Work out the finished part from the listing and answer in its coordinate system (mm). A direction names the side the tool comes from. Round coordinates to 2 decimals unless told otherwise and drop trailing zeros. Order: outer loops, then holes, each group sorted by start corner. A loop starts at its lowest first (then second) coordinate and runs counter-clockwise, first axis right, second up. Notation, with made-up numbers: (-9, 32) - (50, 32) arc R20 cw to (50, 67) - close; hole circle Ø4 at (-23, 75). An arc over 180 degrees is marked (long way). Use one line per item in the form item = value. Start each with the question number.
Q1. The part is cut by section D-D on z = 21.65. Determine the outline of the cut face in (x, y).
Q2. The part is cut by section B-B on y = 14. Determine the outline of the cut face in (x, z), plus the area to 3 significant figures.
Q3. The part is cut by section C-C on x = -15.65. Determine the outline of the cut face in (y, z), plus the area to 4 significant figures.
Q4. Given P1, Ø22.5, axis at x = 15, z = 10, coming from the +Y side; P2, Ø1, axis at x = -21.5, y = 17.5, coming from the +Z side; P3, Ø1.5, axis at x = -20, z = -4.5, coming from the -Y side, each flat-ended and moving along its own axis, determine where each tip first touches the part or whether it passes through.
Q5. Which of the six approach directions +Z, -Z, +X, -X, +Y, -Y give full straight-line access (tool end or side, diameter ignored) to faces 4 (the cylindrical face through (-17, 7, -9)), 5 (the flat face through (0, 35, -16.5))?
Q6. Find the intervals of material crossed by line 1 (Z direction, x = -15.65, y = 10.5); line 2 (X direction, y = 7.5, z = 22); line 3 (X direction, y = 9, z = -9), in increasing order. Write a range as [from, to].
Q7. For a pull along X with two mould halves and no side action, classify faces 1 (the cylindrical face through (15.325, 7.395, 20.186)), 2 (the flat face through (0, 7, 28.5)), 3 (the flat face through (32.5, 9, -7)) as +X half, -X half, draft (parallel to the pull), parting line (faces both ways), or undercut.
Q8. The part is cut by section A-A on z = 6. Determine the outline of the cut face in (x, y), plus the area to 3 significant figures.
from build123d import *

# Parameters (mm, degrees)
F0_W      = 65
F0_H      = 57
F1_DEPTH  = 55
F2_W      = 65
F2_H      = 45
F3_DEPTH  = 40
F4_R      = 11
F5_DEPTH  = 15
F6_R      = 1.5
F10_DEPTH = 15
F7_R      = 1.5
F11_DEPTH = 15
F8_R      = 1.5
F12_DEPTH = 15
F9_R      = 1.5
F13_DEPTH = 15


with BuildPart() as f1:
    # F0 (on Front) → F1 (new body)
    with BuildSketch(Plane.XZ):
        Rectangle(F0_W, F0_H)
    extrude(amount=-F1_DEPTH)

    # F2 (on face) → F3 (cut)
    with BuildSketch(Plane(origin=(0, 55, 0), x_dir=(-1, 0, 0), z_dir=(0, 1, 0))):
        with Locations((0, 6)):
            Rectangle(F2_W, F2_H)
    extrude(amount=-F3_DEPTH, mode=Mode.SUBTRACT)

    # F4 (on face) → F5 (cut)
    with BuildSketch(Plane.XZ):
        with Locations((0, 6)):
            Circle(F4_R)
    extrude(amount=-F5_DEPTH, mode=Mode.SUBTRACT)

    # F6 (on face) → F10 (cut)
    with BuildSketch(Plane.XZ):
        with Locations((15.65, 21.65)):
            Circle(F6_R)
    extrude(amount=-F10_DEPTH, mode=Mode.SUBTRACT)

    # F7 (on face) → F11 (cut)
    with BuildSketch(Plane.XZ):
        with Locations((-15.65, 21.65)):
            Circle(F7_R)
    extrude(amount=-F11_DEPTH, mode=Mode.SUBTRACT)

    # F8 (on face) → F12 (cut)
    with BuildSketch(Plane.XZ):
        with Locations((15.65, -9.65)):
            Circle(F8_R)
    extrude(amount=-F12_DEPTH, mode=Mode.SUBTRACT)

    # F9 (on face) → F13 (cut)
    with BuildSketch(Plane.XZ):
        with Locations((-15.65, -9.65)):
            Circle(F9_R)
    extrude(amount=-F13_DEPTH, mode=Mode.SUBTRACT)


solid = f1.part
Found:
q1.outline = (-32.5, 0) - (-17.15, 0) - (-17.15, 15) - (-32.5, 15) - close; (-14.15, 0) - (14.15, 0) - (14.15, 15) - (-14.15, 15) - close; (17.15, 0) - (32.5, 0) - (32.5, 15) - (17.15, 15) - close
q2.outline = (-32.5, -28.5) - (32.5, -28.5) - (32.5, 28.5) - (-32.5, 28.5) - close; hole circle Ø3 at (-15.65, -9.65); hole circle Ø3 at (-15.65, 21.65); hole circle Ø22 at (0, 6); hole circle Ø3 at (15.65, -9.65); hole circle Ø3 at (15.65, 21.65)
q2.area = 3,300 mm²
q3.outline = (0, -28.5) - (55, -28.5) - (55, -16.5) - (15, -16.5) - (15, -11.15) - (0, -11.15) - close; (0, -8.15) - (15, -8.15) - (15, 20.15) - (0, 20.15) - close; (0, 23.15) - (15, 23.15) - (15, 28.5) - (0, 28.5) - close
q3.area = 1,245 mm²
q4.P1 = 15
q4.P2 = -16.5
q4.P3 = 0
q5.face_4 = +Y, -Y
q5.face_5 = +Z, +X, -X, +Y
q6.line_1 = [-28.5, -11.15], [-8.15, 20.15], [23.15, 28.5]
q6.line_2 = [-32.5, -17.11], [-14.19, 14.19], [17.11, 32.5]
q6.line_3 = [-32.5, -17], [-14.3, 14.3], [17, 32.5]
q7.face_1 = undercut
q7.face_2 = draft
q7.face_3 = +X half
q8.outline = (-32.5, 0) - (-11, 0) - (-11, 15) - (-32.5, 15) - close; (11, 0) - (32.5, 0) - (32.5, 15) - (11, 15) - close
q8.area = 645 mm²
